from build123d import *

# Parameters (mm, degrees)
BASE_EXTRUSION_DEPTH    = 17
CONG_1_R                = 5
CONG_2_R                = 5
CONG_3_R                = 5
CONG_4_R                = 5
ESQUISSE5_R             = 16.5
BOSS_EXTRU_1_DEPTH      = 16
ENL_V_START             = -43.991208
ESQUISSE9_W             = 10.8
ESQUISSE9_H             = 51.405339809
ENL_V_MAT_EXTRU_2_DEPTH = 87.982416
ESQUISSE15_R            = 6
BOSS_EXTRU_2_DEPTH      = 26
ESQUISSE16_R            = 8
BOSS_EXTRU_3_DEPTH      = 19
CHANFREIN1_SIZE         = 1
ESQUISSE17_R            = 1.75
ENL_V_MAT_EXTRU_3_DEPTH = 80.254188527
ESQUISSE18_R            = 11
ENL_V_MAT_EXTRU_4_DEPTH = 12
ESQUISSE19_R            = 4.5
ENL_V_MAT_EXTRU_5_DEPTH = 82
CHANFREIN2_SIZE         = 1
CHANFREIN3_SIZE         = 1
ESQUISSE23_W            = 1.45
ESQUISSE23_H            = 25
EXTRUSION1_START        = -10
EXTRUSION1_DEPTH        = 10


with BuildPart() as part:
    # Esquisse1 → Base-Extrusion (new body)
    with BuildSketch(Plane.XY):
        Polygon((-17, 0), (17, 0), (32.198684154, 5), (45.557198765, 37.350426386), (26, 45), (-26, 45), (-45.557198765, 37.350426386), (-32.198684154, 5), align=None)
    extrude(amount=BASE_EXTRUSION_DEPTH)

    # Congé1
    cong_1_edges = [part.edges().sort_by_distance(p)[0] for p in [
        (45.557198765, 37.350426386, 8.5),
    ]]
    fillet(cong_1_edges, radius=CONG_1_R)

    # Congé2
    cong_2_edges = [part.edges().sort_by_distance(p)[0] for p in [
        (-45.557198765, 37.350426386, 8.5),
    ]]
    fillet(cong_2_edges, radius=CONG_2_R)

    # Congé3
    cong_3_edges = [part.edges().sort_by_distance(p)[0] for p in [
        (-32.198684154, 5, 8.5),
    ]]
    fillet(cong_3_edges, radius=CONG_3_R)

    # Congé4
    cong_4_edges = [part.edges().sort_by_distance(p)[0] for p in [
        (32.198684154, 5, 8.5),
    ]]
    fillet(cong_4_edges, radius=CONG_4_R)

    # Esquisse5 → Boss.-Extru.1 (add)
    with BuildSketch(Plane(origin=(0, 45, 0), x_dir=(-1, 0, 0), z_dir=(0, 1, 0))):
        with Locations(Location((0, 8.5, 0), (0, 0, 211.007583007))):
            Circle(ESQUISSE5_R)
    extrude(amount=BOSS_EXTRU_1_DEPTH)

    # Esquisse9 → Enlèv. mat.-Extru.2 (cut)
    with BuildSketch(Plane(origin=(0, 0, 0), x_dir=(0, 0, -1), z_dir=(1, 0, 0)).offset(ENL_V_START)):
        with Locations((-8.5, 20.378761833)):
            Rectangle(ESQUISSE9_W, ESQUISSE9_H)
    extrude(amount=ENL_V_MAT_EXTRU_2_DEPTH, mode=Mode.SUBTRACT)

    # Esquisse14 → Boss.-Révol.1 (revolve)
    with BuildSketch(Plane(origin=(0, 0, 0), x_dir=(0, 0, -1), z_dir=(1, 0, 0))):
        Polygon((-8.5, 45.740204338), (-22.261709351, 45.740204338), (-13.428527568, 24.827476443), (-8.5, 24.827476443), align=None)
    revolve(axis=Axis((0, 54.838113355, 8.5), (0, -1, 0)))

    # Esquisse15 → Boss.-Extru.2 (add)
    with BuildSketch(Plane.XZ.offset(-24.827476443)):
        with Locations(Location((0, 8.5, 0), (0, 0, 64.158067237))):
            Circle(ESQUISSE15_R)
    extrude(amount=BOSS_EXTRU_2_DEPTH)

    # Esquisse16 → Boss.-Extru.3 (add)
    with BuildSketch(Plane.XZ.offset(1.172523557)):
        with Locations(Location((0, 8.5, 0), (0, 0, 270))):
            Circle(ESQUISSE16_R)
    extrude(amount=BOSS_EXTRU_3_DEPTH)

    # Chanfrein1
    chanfrein1_edges = [part.edges().sort_by_distance(p)[0] for p in [
        (0, -20.172523557, 16.5),
    ]]
    chamfer(chanfrein1_edges, length=CHANFREIN1_SIZE)

    # Esquisse17 → Enlèv. mat.-Extru.3 (cut, through all)
    with BuildSketch(Plane.XY.offset(17)):
        with Locations((-36.5, 37)):
            Circle(ESQUISSE17_R)
        with Locations((-18.5, 37)):
            Circle(ESQUISSE17_R)
        with Locations((-12.5, 10)):
            Circle(ESQUISSE17_R)
        with Locations((12.5, 10)):
            Circle(ESQUISSE17_R)
        with Locations((18.5, 37)):
            Circle(ESQUISSE17_R)
        with Locations((36.5, 37)):
            Circle(ESQUISSE17_R)
    extrude(amount=-ENL_V_MAT_EXTRU_3_DEPTH, mode=Mode.SUBTRACT)

    # Esquisse18 → Enlèv. mat.-Extru.4 (cut)
    with BuildSketch(Plane(origin=(0, 61, 0), x_dir=(-1, 0, 0), z_dir=(0, 1, 0))):
        with Locations(Location((0, 8.5, 0), (0, 0, 90))):
            Circle(ESQUISSE18_R)
    extrude(amount=-ENL_V_MAT_EXTRU_4_DEPTH, mode=Mode.SUBTRACT)

    # Esquisse19 → Enlèv. mat.-Extru.5 (cut)
    with BuildSketch(Plane(origin=(0, 49, 0), x_dir=(-1, 0, 0), z_dir=(0, 1, 0))):
        with Locations(Location((0, 8.5, 0), (0, 0, 90))):
            Circle(ESQUISSE19_R)
    extrude(amount=-ENL_V_MAT_EXTRU_5_DEPTH, mode=Mode.SUBTRACT)

    # Chanfrein2
    chanfrein2_edges = [part.edges().sort_by_distance(p)[0] for p in [
        (0, 61, -2.5),
    ]]
    chamfer(chanfrein2_edges, length=CHANFREIN2_SIZE)

    # Chanfrein3
    chanfrein3_edges = [part.edges().sort_by_distance(p)[0] for p in [
        (-14.142135624, 61, 17),
    ]]
    chamfer(chanfrein3_edges, length=CHANFREIN3_SIZE)

    # Esquisse23 → Trou taraudé M3.5x0.61 (revolve, cut)
    with BuildSketch(Plane(origin=(0, 52, 0), x_dir=(0, 1, 0), z_dir=(1, 0, 0))):
        with Locations((0.725, 12.5)):
            Rectangle(ESQUISSE23_W, ESQUISSE23_H)
    revolve(axis=Axis((0, 52, -6.35), (0, 0, 1)), mode=Mode.SUBTRACT)

    # Esquisse24 → Extrusion1 (cut)
    with BuildSketch(Plane(origin=(0, 61, 0), x_dir=(-1, 0, 0), z_dir=(0, 1, 0)).offset(EXTRUSION1_START)):
        with BuildLine():
            Line((16.431676725, 10), (12.431676725, 10))
            Line((12.431676725, 10), (12.431676725, 7))
            Line((12.431676725, 7), (16.431676725, 7))
            ThreePointArc((16.431676725, 7), (16.5, 8.5), (16.431676725, 10))
        make_face()
    extrude(amount=EXTRUSION1_DEPTH, mode=Mode.SUBTRACT)


solid = part.part
Source: CAD feature listing. Evaluate the final solid. Frame: model axes, mm. A direction names the side the tool comes from. Round coordinates to 2 decimals unless told otherwise and drop trailing zeros. Loops run counter-clockwise (first coordinate to the right, second up) from the corner with the lowest first, then second, coordinate; pieces in that order, holes last.
Q1. Section C-C, the plane y = 1. Return loops of the section in (x, z).
Q2. Ray query, line 1 (Z direction, x = -22.5, y = 38.5); line 2 (Y direction, x = 18.5, z = 2.4); line 3 (Z direction, x = -4, y = 12). Return the intervals inside material, ascending.
Q3. Section B-B, the plane x = -18.5. Return loops of the section in (y, z), plus the area to 3 significant figures.
Q4. First-contact query: P1, Ø1.6, axis at x = -17.5, z = 15, coming from the +Y side; P2, Ø4, axis at x = 1, z = -6, coming from the -Y side; P3, Ø8, axis at x = -3, z = 10, coming from the +Y side. Flat tips, straight axial feed; report the tip coordinate or a pass-through.
Q5. Mould query, pull axis X, two halves, no side actions, for faces 4 (the face through (-14, 56, 10)), 5 (the face through (-38.418, 20.061, 15.428)), 6 (the face through (-18.88, 35.29, 1.57)). Classes: pulls with the +X half, pulls with the -X half, needs draft (parallel to the pull), parting line crosses it, or undercut.
Q6. Access query for faces 1 (the face through (-34.883, 36.33, 1.572)), 2 (the face through (-5, 24.827, 10)), 3 (the face through (-5, 49, 8)). Directions: +Z, -Z, +X, -X, +Y, -Y. A direction counts if a zero-diameter tool reaches every point of the face in a straight line with its end or side. Return the directions, or none.
Q7. Section A-A, the plane y = 10. State how many separate pieces and enclosed holes the cut face has, plus the area to 3 significant figures.
Solutions:
1. outline: (-20.04, 0) - (20.04, 0) - (20.04, 3.1) - (2.62, 3.1) arc R6 ccw to (2.62, 13.9) - (20.04, 13.9) - (20.04, 17) - (-20.04, 17) - (-20.04, 13.9) - (-2.62, 13.9) arc R6 ccw to (-2.62, 3.1) - (-20.04, 3.1) - close; hole circle Ø9 at (0, 8.5)
2. line 1: z = 0 to 3.1, 13.9 to 17
2. line 2: y = 0.49 to 35.25, 38.75 to 45
2. line 3: z = 0 to 3.1, 4.03 to 6.44, 10.56 to 12.97, 13.9 to 17
3. outline: (0.49, 0) - (35.25, 0) - (35.25, 3.1) - (0.49, 3.1) - close; (0.49, 13.9) - (35.25, 13.9) - (35.25, 17) - (0.49, 17) - close; (38.75, 0) - (45, 0) - (45, 3.1) - (38.75, 3.1) - close; (38.75, 13.9) - (45, 13.9) - (45, 17) - (38.75, 17) - close
3. area: 254 mm2
4. P1: stops at y = 45
4. P2: stops at y = 42.83
4. P3: stops at y = 49
5. face 4: needs draft
5. face 5: pulls with the -X half
5. face 6: undercut
6. face 1: +Z, -Z
6. face 2: none
6. face 3: +Y
7. separate pieces: 5
7. enclosed holes: 1
7. area: 427 mm2
